```python
from build123d import *

# Parameters (mm, degrees)
SKETCH_2_W               = 200
SKETCH_2_H               = 50
EXTRUDE_1_DEPTH          = 160
SHELL_1_T                = -5
M8X1_0_1_D               = 8
M8X1_0_1_CSINK_D         = 8.05
M8X1_0_1_CSINK_ANGLE     = 100
PATTERN_CIRCULAR_1_COUNT = 8


with BuildPart() as part:
    # 草图2 → 凸台-拉伸1 (new body)
    with BuildSketch(Plane.XY):
        with Locations((-100, 25)):
            Rectangle(SKETCH_2_W, SKETCH_2_H)
    extrude(amount=EXTRUDE_1_DEPTH)

    # 抽壳1
    shell_1_openings = [part.faces().sort_by_distance(p)[0] for p in [
        (-100, 50, 80),
    ]]
    offset(amount=SHELL_1_T, openings=shell_1_openings, kind=Kind.INTERSECTION)

    # M8x1.0 螺纹孔1 (through all)
    with Locations(Plane(origin=(0, 5, 0), x_dir=(1, 0, 0), z_dir=(0, 1, 0))):
        with Locations((-80, -40)):
            m8x1_0_1 = CounterSinkHole(M8X1_0_1_D / 2, M8X1_0_1_CSINK_D / 2, counter_sink_angle=M8X1_0_1_CSINK_ANGLE)

    # 阵列(圆周)1: M8x1.0 螺纹孔1 ×8 about axis
    pattern_circular_1_axis = Axis((-80, 0, 80), (0, 1, 0))
    for i in range(1, PATTERN_CIRCULAR_1_COUNT):
        add(m8x1_0_1.rotate(pattern_circular_1_axis, i * 360 / PATTERN_CIRCULAR_1_COUNT), mode=Mode.SUBTRACT)


solid = part.part
```
Can you work these out from the model? Positions are in its coordinate system, mm. A direction names the side the tool comes from. Coordinates: 2 decimals unless noted, no trailing zeros. Loops run counter-clockwise (first coordinate to the right, second up) from the corner with the lowest first, then second, coordinate; pieces in that order, holes last. Notation, with made-up numbers: (-5, -12) - (28, -12) arc R12 cw to (28, 10) - close; hole circle Ø6 at (-22.75, 35.25). An arc over 180 degrees is marked (long way). Use a Markdown table: item, result.
Item 1: I want a section at A-A on y = 12.5. Please give me the cut outline in (x, z).
Numbers:
| item | result |
|---|---|
| outline | (-200, 0) - (0, 0) - (0, 160) - (-200, 160) - close; hole (-195, 5) - (-5, 5) - (-5, 155) - (-195, 155) - close |
Item 2: I want a section at D-D on z = 120. Please give me the cut outline in (x, y) (3 decimals).
Numbers:
| item | result |
|---|---|
| outline | (-200, 0) - (-84, 0) - (-84, 4.979) - (-84.025, 5) - (-195, 5) - (-195, 50) - (-200, 50) - close; (-76, 0) - (0, 0) - (0, 50) - (-5, 50) - (-5, 5) - (-75.975, 5) - (-76, 4.979) - close |
Item 3: Will this pin go through, and if not, where does the flat tip stop? pin 1 (5 mm diameter, centred on x = -151, z = 96.5, fed in from +Y).
Numbers:
| item | result |
|---|---|
| pin 1 | stops at y = 5 |
Item 4: I want a section at C-C on z = 80. Please give me the cut outline in (x, y) (3 decimals).
Numbers:
| item | result |
|---|---|
| outline | (-200, 0) - (-124, 0) - (-124, 4.979) - (-124.025, 5) - (-195, 5) - (-195, 50) - (-200, 50) - close; (-116, 0) - (-44, 0) - (-44, 4.979) - (-44.025, 5) - (-115.975, 5) - (-116, 4.979) - close; (-36, 0) - (0, 0) - (0, 50) - (-5, 50) - (-5, 5) - (-35.975, 5) - (-36, 4.979) - close |
Item 5: We'd pull the mould along Z, two halves only. Please class faces 3 (the face through (-112.28, 2.45, 108.11)), 4 (the face through (-101, 25, 160)), 5 (the face through (-200, 25, 79)), 6 (the face through (-101, 25, 0)): released by +Z, released by -Z, zero draft, split by the parting line, or undercut.
Numbers:
| item | result |
|---|---|
| face 3 | undercut |
| face 4 | released by +Z |
| face 5 | zero draft |
| face 6 | released by -Z |
Item 6: I want a section at B-B on x = -120. Please give me the cut outline in (y, z) (3 decimals).
Numbers:
| item | result |
|---|---|
| outline | (0, 0) - (50, 0) - (50, 5) - (5, 5) - (5, 75.975) - (4.979, 76) - (0, 76) - close; (0, 84) - (4.979, 84) - (5, 84.025) - (5, 155) - (50, 155) - (50, 160) - (0, 160) - close |
Item 7: If I drill on probe 1 along X at (y, z) = (40.5, 137); probe 2 along Z at (x, y) = (-158, 31.5); probe 3 along Z at (x, y) = (-50.5, 3), over which ranges is the centre line in solid material (lowest first)? Write a range as from..to.
Numbers:
| item | result |
|---|---|
| probe 1 | x = -200..-195, -5..0 |
| probe 2 | z = 0..5, 155..160 |
| probe 3 | z = 0..47.9, 55.53..104.47, 112.1..160 |
Item 8: For faces 1 (the face through (-80.521, 2.455, 123.966)), 2 (the face through (-101, 28, 5)), which set-ups out of +Z, -Z, +X, -X, +Y, -Y let a thin tool reach every point of the face, with its end or its side?
Numbers:
| item | result |
|---|---|
| face 1 | +Y, -Y |
| face 2 | +Y |
